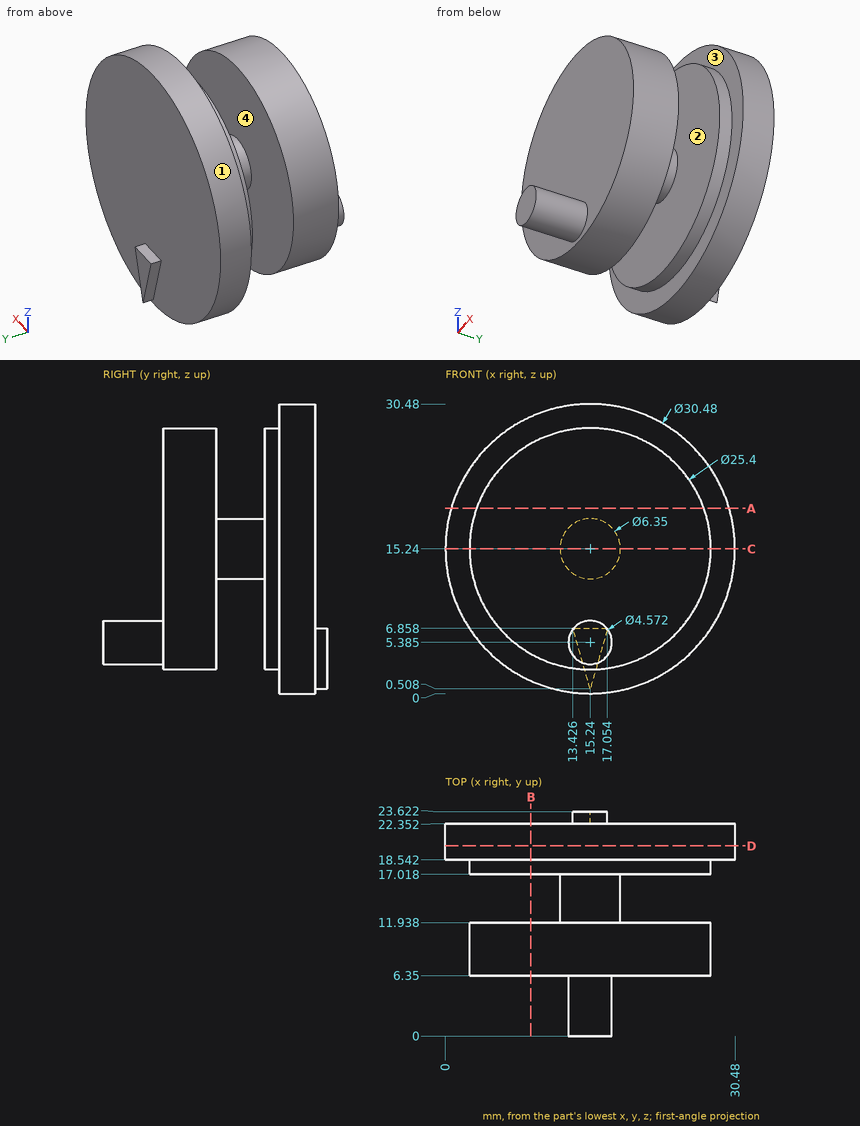
Could you check a few things on this drawing? It's one solid part, dimensions in mm from its lowest x, y, z. Coordinates: 2 decimals unless noted, no trailing zeros. Order: outer loops, then holes, each group sorted by start corner. A loop starts at its lowest first (then second) coordinate and runs counter-clockwise, first axis right, second up.
1) Will these pins go through, and if not, where does the flat tip stop? pin 1 (6 mm diameter, centred on x = 12.5, z = 22.5, fed in from +Y); pin 2 (4 mm diameter, centred on x = 22.5, y = 16, fed in from +Z); pin 3 (12.5 mm diameter, centred on x = 18, z = 16.5, fed in from -Y).
2) Imagine slicing it at D-D on y = 20. List the corners of the cut face in (x, z) for me.
3) Imagine slicing it at C-C on z = 15.24. List the corners of the cut face in (x, y) for me (3 decimals), and give its area (3 significant figures).
4) Imagine slicing it at B-B on x = 9. List the corners of the cut face in (y, z) for me.
5) We'd pull the mould along Y, two halves only. Please class the marked faces 1, 2, 3 and 4: +Y half, -Y half, draft (parallel to the pull), parting line (faces both ways), or undercut.
6) Imagine slicing it at A-A on z = 19.5. List the corners of the cut face in (x, y) for me, and give its area (3 significant figures).
7) I need wall thicknesses on line 1 (Y direction, x = 21, z = 18); line 2 (Z direction, x = 15, y = 15.75). Which ranges of each line are inside material? Lowest first, please.
Response values:
1. pin 1: stops at y = 22.35
1. pin 2: stops at z = 26.67
1. pin 3: stops at y = 6.35
2. outline: circle Ø30.48 at (15.24, 15.24)
3. outline: (0, 18.542) - (2.54, 18.542) - (2.54, 17.018) - (12.065, 17.018) - (12.065, 11.938) - (2.54, 11.938) - (2.54, 6.35) - (27.94, 6.35) - (27.94, 11.938) - (18.415, 11.938) - (18.415, 17.018) - (27.94, 17.018) - (27.94, 18.542) - (30.48, 18.542) - (30.48, 22.352) - (0, 22.352) - close
3. area: 329 mm2
4. outline: (6.35, 4.18) - (11.94, 4.18) - (11.94, 26.3) - (6.35, 26.3) - close; (17.02, 4.18) - (18.54, 4.18) - (18.54, 1.34) - (22.35, 1.34) - (22.35, 29.14) - (18.54, 29.14) - (18.54, 26.3) - (17.02, 26.3) - close
5. face 1: draft
5. face 2: undercut
5. face 3: -Y half
5. face 4: undercut
6. outline: (0.61, 18.54) - (3.28, 18.54) - (3.28, 17.02) - (27.2, 17.02) - (27.2, 18.54) - (29.87, 18.54) - (29.87, 22.35) - (0.61, 22.35) - close; (3.28, 6.35) - (27.2, 6.35) - (27.2, 11.94) - (3.28, 11.94) - close
6. area: 282 mm2
7. line 1: y = 6.35 to 11.94, 17.02 to 22.35
7. line 2: z = 12.07 to 18.41
